Check sheet for the modelled part. Datum: model origin and axes. Units: mm. Face numbers are marked on the shaded views. A direction names the side the tool comes from. Round coordinates to 2 decimals unless told otherwise and drop trailing zeros. Loops run counter-clockwise (first coordinate to the right, second up) from the corner with the lowest first, then second, coordinate; pieces in that order, holes last. Notation, with made-up numbers: M 59,60 L 73,60 A22 cw 73,81 Z; hole C 83,-17 d4. An arc over 180 degrees is marked long. Write item = value, one per line. Start each with the question number.
(1) Scan lines: L1, parallel to Y at x = -15.5, z = 12; L2, parallel to Y at x = 6.5, z = 61; L3, parallel to Y at x = -18.5, z = 47.5. Record each from-to range of solid material in increasing order. Write a range as from..to.
(2) Mould release check, pull along X, two halves, no side actions. Record for the marked faces 1, 2 and 3: pulls with the +X half, pulls with the -X half, needs draft (parallel to the pull), parting line crosses it, or undercut.
(3) Cross-section at B-B on z = 24. Record the boundary of the cut face in (x, y), plus the area to 4 significant figures.
(4) Cross-section at C-C on y = -3. Record the boundary of the cut face in (x, z).
(5) Go/stop test with flat-tipped pins: P1, Ø17.5, axis at y = -7.5, z = 66, coming from the -X side; P2, Ø13.5, axis at y = -230, z = 51, coming from the +X side; P3, Ø22.5, axis at y = -219.5, z = 43, coming from the -X side. Record where each tip stops, or that it passes through.
(6) Cross-section at A-A on x = 9. Record the boundary of the cut face in (y, z), plus the area to 3 significant figures.
(7) Set-up check for the marked faces 4, 5, 6, 7 and 8: record each of +Z, -Z, +X, -X, +Y, -Y from which the full face is reachable in a straight line by a thin tool's end or side.
(8) Cross-section at D-D on x = -38.5. Record the boundary of the cut face in (y, z).
from build123d import *

# Parameters (mm, degrees)
ESQUISSE2_W        = 40
ESQUISSE2_H        = 40
ESQUISSE2_W_2      = 35
ESQUISSE2_H_2      = 35
BOSS_EXTRU_1_DEPTH = 100
ESQUISSE3_W        = 25
ESQUISSE3_H        = 45
BOSS_EXTRU_2_DEPTH = 300
ESQUISSE4_W        = 100
ESQUISSE4_H        = 100
BOSS_EXTRU_3_DEPTH = 25


with BuildPart() as part:
    # Esquisse2 → Boss.-Extru.1 (new body)
    with BuildSketch(Plane.XY):
        Rectangle(ESQUISSE2_W, ESQUISSE2_H)
        Rectangle(ESQUISSE2_W_2, ESQUISSE2_H_2, mode=Mode.SUBTRACT)
    extrude(amount=BOSS_EXTRU_1_DEPTH)

    # Esquisse3 → Boss.-Extru.2 (add)
    with BuildSketch(Plane.XZ.offset(20)):
        with Locations((0, 50)):
            Rectangle(ESQUISSE3_W, ESQUISSE3_H)
    extrude(amount=BOSS_EXTRU_2_DEPTH)

    # Esquisse4 → Boss.-Extru.3 (add)
    with BuildSketch(Plane.XZ.offset(320)):
        with Locations((0, 50)):
            Rectangle(ESQUISSE4_W, ESQUISSE4_H)
    extrude(amount=BOSS_EXTRU_3_DEPTH)


solid = part.part
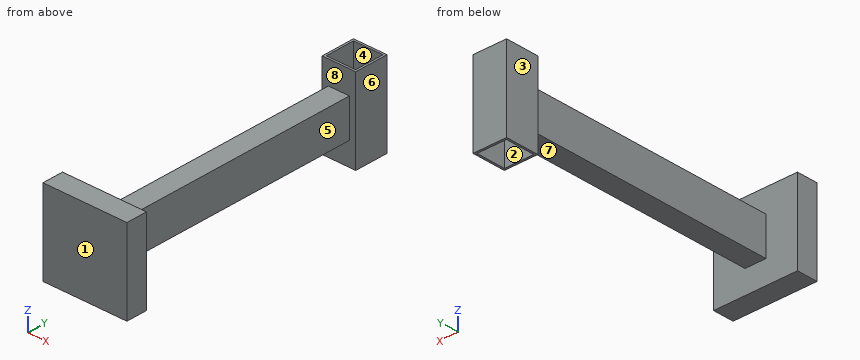
Result:
q1.L1 = -345..-320, -20..-17.5, 17.5..20
q1.L2 = -345..-17.5, 17.5..20
q1.L3 = -345..-320, -20..20
q2.face_1 = needs draft
q2.face_2 = undercut
q2.face_3 = pulls with the -X half
q3.outline = M -50,-345 L 50,-345 L 50,-320 L -50,-320 Z; M -20,-20 L 20,-20 L 20,20 L -20,20 Z; hole M -17.5,-17.5 L 17.5,-17.5 L 17.5,17.5 L -17.5,17.5 Z
q3.area = 2,875 mm^2
q4.outline = M -20,0 L -17.5,0 L -17.5,100 L -20,100 Z; M 17.5,0 L 20,0 L 20,100 L 17.5,100 Z
q5.P1 = -20
q5.P2 = 12.5
q5.P3 = -12.5
q6.outline = M -345,0 L -320,0 L -320,27.5 L -20,27.5 L -20,0 L -17.5,0 L -17.5,100 L -20,100 L -20,72.5 L -320,72.5 L -320,100 L -345,100 Z; M 17.5,0 L 20,0 L 20,100 L 17.5,100 Z
q6.area = 16,500 mm^2
q7.face_4 = +Z, -Z
q7.face_5 = +Z, -Z, +X
q7.face_6 = +Z, -Z, +X, +Y
q7.face_7 = -Z, +X, -X
q7.face_8 = none
q8.outline = M -345,0 L -320,0 L -320,100 L -345,100 Z
